Geometry check sheet. Reference: the model listing, model coordinates, mm. A direction names the side the tool comes from. Coordinates: 2 decimals unless noted, no trailing zeros. Write each loop counter-clockwise with the first axis right and the second up, starting at its lowest first coordinate (ties: lowest second). Pieces come first, ordered by that corner, then holes. Notation, with made-up numbers: (89.5, 41) -> (103.5, 41) arc R38 ccw to (103.5, 80) -> close; hole circle Ø7 at (-10.75, -9.75). An arc over 180 degrees is marked (long way). Answer in a Markdown table with one row per item. Add a question column.
1. Cross-section at D-D on x = -11.5. Record the cut outline in (y, z) (1 decimal), and give its area (3 significant figures).
2. Cross-section at B-B on z = 1. Give the number of separate pieces and of enclosed holes in the cut face, and give its area (3 significant figures).
3. Mould release check, pull along X, two halves, no side actions. Record for faces 1 (the flat face through (-15, 1, 2.54)), 2 (the cylindrical face through (-4.997, 12.525, 15.869)), 3 (the flat face through (-6, 0, 0)): pulls with the +X half, pulls with the -X half, needs draft (parallel to the pull), parting line crosses it, or undercut.
4. Set-up check for faces 4 (the cylindrical face through (-0.274, -1.127, -14.094)), 5 (the flat face through (7.366, 9, 0)), 6 (the flat face through (-15, 1, -2.54)), 7 (the flat face through (15, 5.207, 0)): record each of +Z, -Z, +X, -X, +Y, -Y from which the full face is reachable in a straight line by a thin tool's end or side.
5. Cross-section at A-A on y = 13.5. Record the cut outline in (x, z), and give its area (3 significant figures).
6. Scan lines: L1, parallel to X at y = 14, z = -7; L2, parallel to Z at x = -4, y = 8; L3, parallel to Z at x = -5, y = 5.25. Record each from-to range of solid material in increasing order. Write a range as from..to.
7. Depth check by flat-ended pin: P1, Ø2, axis at x = -1.5, y = 4.5, coming from the -Z side; P2, Ø4.5, axis at x = -14, z = -1, coming from the -Y side; P3, Ø4, axis at x = 4.5, y = 13.5, coming from the -Z side; P4, Ø0.7, axis at x = 13.5, y = 8, coming from the +Z side. Enter the tip coordinate at first touch or a pass-through.
8. Cross-section at C-C on y = 8. Record the cut outline in (x, z).
```python
from build123d import *

# Parameters (mm, degrees)
SKETCH1_R           = 16.637
SKETCH1_W           = 10.16
SKETCH1_H           = 12.065
BOSS_EXTRUDE1_DEPTH = 15.875
SHELL1_T            = -2.286
BOSS_EXTRUDE2_DEPTH = 1.5875
SKETCH3_W           = 1.5875
SKETCH3_H           = 5.08
BOSS_EXTRUDE3_DEPTH = 13.589
SKETCH7_R           = 16.637
SKETCH7_R_2         = 14.097
BOSS_EXTRUDE4_DEPTH = 2.286
CUT_EXTRUDE1_DEPTH  = 7.493
CUT_EXTRUDE2_DEPTH  = 5.588
CIRPATTERN2_COUNT   = 2
SKETCH6_W           = 1.5875
SKETCH6_H           = 2.286


with BuildPart() as part:
    # Sketch1 → Boss-Extrude1 (new body)
    with BuildSketch(Plane(origin=(0, 0, 0), x_dir=(1, 0, 0), z_dir=(0, 1, 0))):
        with Locations(Location((0, 0, 0), (0, 0, 270))):
            Circle(SKETCH1_R)
        Rectangle(SKETCH1_W, SKETCH1_H, mode=Mode.SUBTRACT)
    extrude(amount=BOSS_EXTRUDE1_DEPTH)

    # Shell1
    shell1_openings = [part.faces().sort_by_distance(p)[0] for p in [
        (0, 15.875, -16.166434579),
    ]]
    offset(amount=SHELL1_T, openings=shell1_openings, kind=Kind.INTERSECTION)

    # Sketch2 → Boss-Extrude2 (add)
    with BuildSketch(Plane.XZ):
        Polygon((-5.08, 6.0325), (-1.905, 6.0325), (-5.08, 2.8575), align=None)
        Polygon((5.08, -2.8575), (1.905, -6.0325), (5.08, -6.0325), align=None)
    extrude(amount=-BOSS_EXTRUDE2_DEPTH)

    # Sketch3 → Boss-Extrude3 (add)
    with BuildSketch(Plane(origin=(0, 15.875, 0), x_dir=(1, 0, 0), z_dir=(0, 1, 0))):
        with Locations((-13.55725, 0)):
            Rectangle(SKETCH3_W, SKETCH3_H)
    boss_extrude3 = extrude(amount=-BOSS_EXTRUDE3_DEPTH)

    # Sketch7 → Boss-Extrude4 (add)
    with BuildSketch(Plane.XZ):
        with Locations(Location((0, 0, 0), (0, 0, 270))):
            Circle(SKETCH7_R)
        with Locations(Location((0, 0, 0), (0, 0, 270))):
            Circle(SKETCH7_R_2, mode=Mode.SUBTRACT)
    extrude(amount=BOSS_EXTRUDE4_DEPTH)

    # Sketch4 → Cut-Extrude1 (cut)
    with BuildSketch(Plane.XZ.offset(2.286)):
        with BuildLine():
            Line((-16.44196366, -2.54), (-12.7635, -2.54))
            Line((-12.7635, -2.54), (-12.7635, 2.54))
            Line((-12.7635, 2.54), (-16.44196366, 2.54))
            ThreePointArc((-16.44196366, 2.54), (-16.637, 0), (-16.44196366, -2.54))
        make_face()
    cut_extrude1 = extrude(amount=-CUT_EXTRUDE1_DEPTH, mode=Mode.SUBTRACT)

    # Sketch5 → Cut-Extrude2 (cut)
    with BuildSketch(Plane(origin=(0, 15.875, 0), x_dir=(1, 0, 0), z_dir=(0, 1, 0))):
        with BuildLine():
            Line((-14.124432767, -2.54), (-12.7635, -2.54))
            Line((-12.7635, -2.54), (-12.7635, 2.54))
            Line((-12.7635, 2.54), (-14.124432767, 2.54))
            ThreePointArc((-14.124432767, 2.54), (-14.351, 0), (-14.124432767, -2.54))
        make_face()
    cut_extrude2 = extrude(amount=-CUT_EXTRUDE2_DEPTH, mode=Mode.SUBTRACT)

    # CirPattern2: Boss-Extrude3, Cut-Extrude1, Cut-Extrude2 ×2 about axis
    cirpattern2_axis = Axis((0, 0, 0), (0, 1, 0))
    add([boss_extrude3.rotate(cirpattern2_axis, i * 360 / CIRPATTERN2_COUNT) for i in range(1, CIRPATTERN2_COUNT)])
    add([cut_extrude1.rotate(cirpattern2_axis, i * 360 / CIRPATTERN2_COUNT) for i in range(1, CIRPATTERN2_COUNT)], mode=Mode.SUBTRACT)
    add([cut_extrude2.rotate(cirpattern2_axis, i * 360 / CIRPATTERN2_COUNT) for i in range(1, CIRPATTERN2_COUNT)], mode=Mode.SUBTRACT)

    # Sketch6 → Revolve1 (revolve)
    with BuildSketch(Plane.XY, mode=Mode.PRIVATE) as revolve1_sk:
        with Locations((-17.43075, 7.9375)):
            Rectangle(SKETCH6_W, SKETCH6_H)
    revolve(revolve1_sk.sketch.rotate(Axis((0, 0, 0), (0, 1, 0)), 188.781790598), axis=Axis((0, 0, 0), (0, 1, 0)))


solid = part.part
```
Results found:
| question | item | result |
|---|---|---|
| 1 | outline | (-2.3, -12) -> (6.8, -12) -> (6.8, -14.1) -> (9.1, -14.1) -> (9.1, -12) -> (15.9, -12) -> (15.9, -8.6) -> (2.3, -8.6) -> (2.3, 8.6) -> (15.9, 8.6) -> (15.9, 12) -> (9.1, 12) -> (9.1, 14.1) -> (6.8, 14.1) -> (6.8, 12) -> (-2.3, 12) -> (-2.3, 8.2) -> (0, 8.2) -> (0, -8.2) -> (-2.3, -8.2) -> close |
| 1 | area | 176 mm^2 |
| 2 | separate pieces | 4 |
| 2 | enclosed holes | 0 |
| 2 | area | 169 mm^2 |
| 3 | face 1 | needs draft |
| 3 | face 2 | parting line crosses it |
| 3 | face 3 | undercut |
| 4 | face 4 | -Y |
| 4 | face 5 | +Y |
| 4 | face 6 | -X, -Y |
| 4 | face 7 | +X, -Y |
| 5 | outline | circle Ø33.27 at (0, 0); (-7.37, -8.32) -> (7.37, -8.32) -> (7.37, 8.32) -> (-7.37, 8.32) -> close; hole circle Ø28.7 at (0, 0); hole (-5.08, -6.03) -> (5.08, -6.03) -> (5.08, 6.03) -> (-5.08, 6.03) -> close |
| 5 | area | 345 mm^2 |
| 6 | L1 | x = -15.09..-12.53, -7.37..7.37, 12.53..15.09 |
| 6 | L2 | z = -17.78..-13.78, -8.32..-6.03, 6.03..8.32, 13.78..17.78 |
| 6 | L3 | z = -15.87..-13.45, -8.32..-6.03, 6.03..8.32, 13.45..15.87 |
| 7 | P1 | stops at z = -16.63 |
| 7 | P2 | stops at y = -2.29 |
| 7 | P3 | stops at z = -16.45 |
| 7 | P4 | stops at z = 12.62 |
| 8 | outline | circle Ø36.45 at (0, 0); (-7.37, -8.32) -> (7.37, -8.32) -> (7.37, 8.32) -> (-7.37, 8.32) -> close; hole (-14.12, -2.54) arc R14.35 ccw to (14.12, -2.54) -> (12.76, -2.54) -> (12.76, 2.54) -> (14.12, 2.54) arc R14.35 ccw to (-14.12, 2.54) -> (-12.76, 2.54) -> (-12.76, -2.54) -> close; hole (-5.08, -6.03) -> (5.08, -6.03) -> (5.08, 6.03) -> (-5.08, 6.03) -> close |
